Geometry check sheet. Reference: drawing and pictorial views, mm from the part's lowest x, y, z. Coordinates: 2 decimals unless noted, no trailing zeros. Loops run counter-clockwise (first coordinate to the right, second up) from the corner with the lowest first, then second, coordinate; pieces in that order, holes last. Notation, with made-up numbers: (-25.5, 37.25) -> (-8.5, 37.25) arc R25 ccw to (-8.5, 73.25) -> close; hole circle Ø11 at (6, 84). An arc over 180 degrees is marked (long way). Answer as a JSON object with one key per item and string values. Group by question number.
Q1. Release check for a two-part mould opening along Y. For the marked faces 1, 2 and 3 record: released by +Y, released by -Y, zero draft, split by the parting line, or undercut.
Q2. Gauge pin test, flat end, axial feed: pin 1 Ø2 at (x, y) = (4.04, 3.5) entering from -Z. Record the tip position at first contact, or that the pin passes through.
Q3. Cross-section at A-A on z = 0.55. Record the boundary of the cut face in (x, y).
Q4. Scan lines: L1, parallel to Y at x = 3.75, z = 0.25 (1 decimal); L2, parallel to Y at x = 4.75, z = 1.3; L3, parallel to X at y = 4.5, z = 0.55 (1 decimal). Record each from-to range of solid material in increasing order.
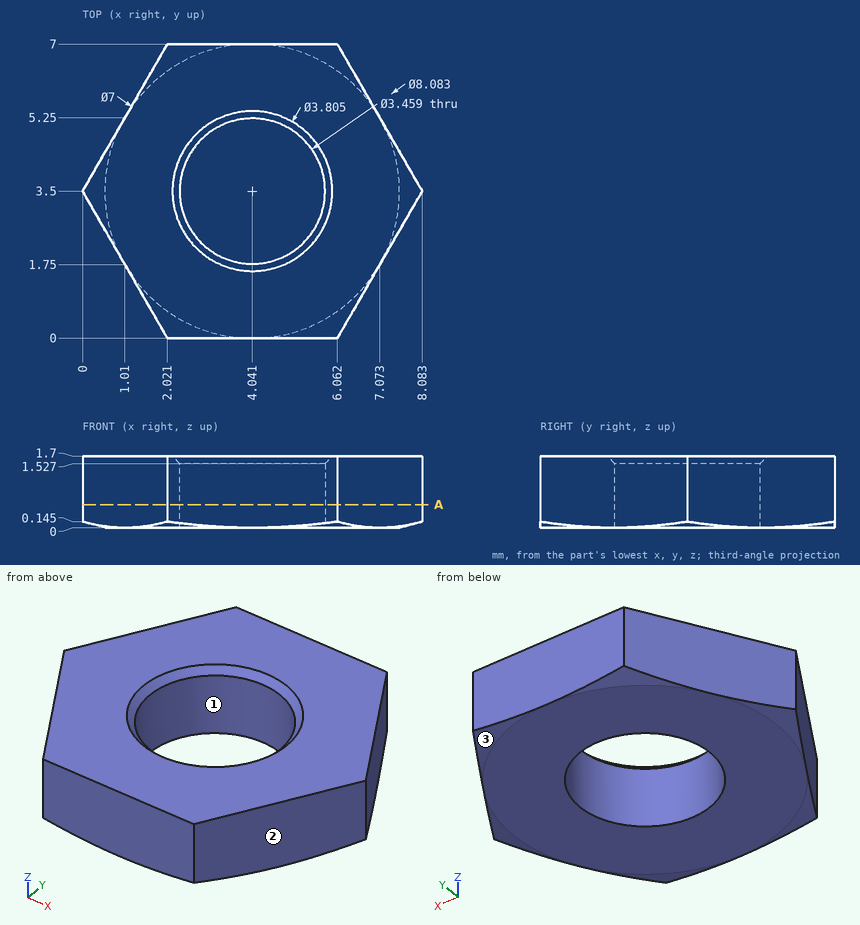
Computed values:
{
 "1": {"face 1": "undercut", "face 2": "released by -Y", "face 3": "released by +Y"},
 "2": {"pin 1": "passes through"},
 "3": {"outline": "(0, 3.5) -> (2.02, 0) -> (6.06, 0) -> (8.08, 3.5) -> (6.06, 7) -> (2.02, 7) -> close; hole circle Ø3.46 at (4.04, 3.5)"},
 "4": {"L1": "y = 0 to 1.8, 5.2 to 7", "L2": "y = 0 to 1.92, 5.08 to 7", "L3": "x = 0.6 to 2.6, 5.5 to 7.5"}
}
